The listing builds one solid part. Answer for the finished solid, in the listing's coordinates (mm). Face numbers are marked on the shaded views. A direction names the side the tool comes from. Give positions to 0.01 mm unless a question says otherwise; leave off trailing zeros. Write each loop counter-clockwise with the first axis right and the second up, starting at its lowest first coordinate (ties: lowest second). Pieces come first, ordered by that corner, then holes. Notation, with made-up numbers: (64.25, 42) -> (80.25, 42) arc R16 cw to (80.25, 69) -> close; hole circle Ø11 at (57, 29.25). An arc over 180 degrees is marked (long way). Write each question's results on one line, items separated by ' | '. Start each with the question number.
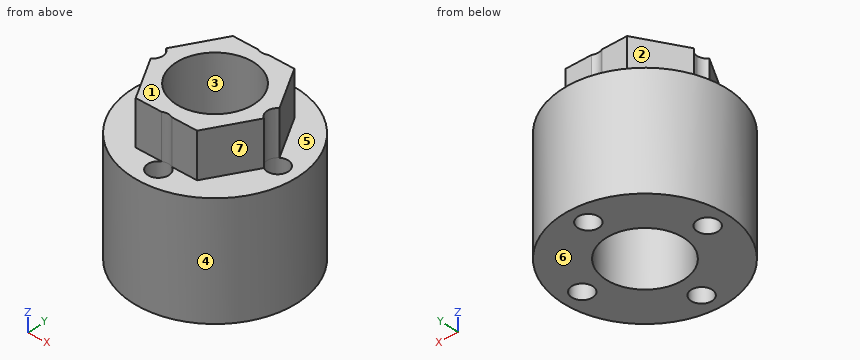
from build123d import *

# Parameters (mm, degrees)
F0_R          = 11
F1_DEPTH      = 15.2
F2_R          = 5.1
F3_DEPTH      = 50
F3_DEPTH_BACK = 50
F4_R          = 1.4
F5_DEPTH      = 25
F7_DEPTH      = 6
F8_R          = 5.2
F9_DEPTH      = 50
F10_DEPTH     = 25


with BuildPart() as f1:
    # F0 (on Top) → F1 (new body)
    with BuildSketch(Plane.XY):
        Circle(F0_R)
    extrude(amount=F1_DEPTH)

    # F2 (on face) → F3 (cut, two sides)
    with BuildSketch(Plane.XY.offset(15.2)) as f3_sk:
        Circle(F2_R)
    extrude(amount=-F3_DEPTH, mode=Mode.SUBTRACT)
    extrude(f3_sk.sketch, amount=-F3_DEPTH_BACK, mode=Mode.SUBTRACT)

    # F4 (on face) → F5 (cut)
    with BuildSketch(Plane.XY.offset(15.2)):
        with Locations((0, -8.3)):
            Circle(F4_R)
        with Locations((-8.3, 0)):
            Circle(F4_R)
        with Locations((0, 8.3)):
            Circle(F4_R)
        with Locations((8.3, 0)):
            Circle(F4_R)
    extrude(amount=-F5_DEPTH, mode=Mode.SUBTRACT)

    # F6 (on face) → F7 (join)
    with BuildSketch(Plane.XY.offset(15.2)):
        Polygon((4.039756, -7.100789), (8.169342, -0.051863), (4.129585, 7.048926), (-4.039756, 7.100789), (-8.169342, 0.051863), (-4.129585, -7.048926), align=None)
    extrude(amount=F7_DEPTH)

    # F8 (on face) → F9 (cut)
    with BuildSketch(Plane.XY.offset(21.2)):
        Circle(F8_R)
    extrude(amount=-F9_DEPTH, mode=Mode.SUBTRACT)

    # F4 (on face) → F10 (cut)
    with BuildSketch(Plane.XY.offset(15.2)):
        with Locations((-8.3, 0)):
            Circle(F4_R)
        with Locations((8.3, 0)):
            Circle(F4_R)
        with Locations((0, 8.3)):
            Circle(F4_R)
        with Locations((0, -8.3)):
            Circle(F4_R)
    extrude(amount=F10_DEPTH, mode=Mode.SUBTRACT)


solid = f1.part
1. Section B-B (z = 18) is taken. Write down the section's boundary in (x, y).
2. The mould has two halves that part along X. Classify the marked faces 1, 2, 3 and 4: pulls with the +X half, pulls with the -X half, needs draft (parallel to the pull), parting line crosses it, or undercut.
3. Section A-A (x = 0) is taken. Write down the section's boundary in (y, z).
4. Consider probe 1 along Y at (x, z) = (0, 5.25); probe 2 along Y at (x, z) = (0.5, 13); probe 3 along Z at (x, y) = (-7.5, 2.75). Determine where each line is inside the solid, lowest interval first. Write a range as [from, to].
5. Section C-C (y = 8.3) is taken. Write down the section's boundary in (x, z).
6. A tool of negligible diameter and unlimited length cuts with its end or side. For the marked faces 5, 6 and 7, from which of +Z, -Z, +X, -X, +Y, -Y can it reach the whole face along a straight path? Write none if from no direction.
7. Each of these flat-tipped pins is pushed along its axis until it touches: pin 1 Ø3 at (y, z) = (3.5, 6.5) entering from -X; pin 2 Ø2 at (y, z) = (2, 8.5) entering from -X; pin 3 Ø3 at (y, z) = (-6.5, 13) entering from -X. Where does it stop, or does it pass through?
8. Section D-D (z = 9.5) is taken. Write down the section's boundary in (x, y), then the cut area to 3 significant figures.
Results:
1) outline: (-7.52, 1.16) arc R1.4 cw to (-7.49, -1.14) -> (-4.13, -7.05) -> (-0.67, -7.07) arc R1.4 cw to (0.69, -7.08) -> (4.04, -7.1) -> (7.52, -1.16) arc R1.4 cw to (7.49, 1.14) -> (4.13, 7.05) -> (0.67, 7.07) arc R1.4 cw to (-0.69, 7.08) -> (-4.04, 7.1) -> close; hole circle Ø10.4 at (0, 0)
2) face 1: needs draft | face 2: pulls with the -X half | face 3: undercut | face 4: parting line crosses it
3) outline: (-11, 0) -> (-9.7, 0) -> (-9.7, 15.2) -> (-11, 15.2) -> close; (-6.9, 0) -> (-5.2, 0) -> (-5.2, 21.2) -> (-6.9, 21.2) -> close; (5.2, 0) -> (6.9, 0) -> (6.9, 21.2) -> (5.2, 21.2) -> close; (9.7, 0) -> (11, 0) -> (11, 15.2) -> (9.7, 15.2) -> close
4) probe 1: y = [-11, -9.7], [-6.9, -5.2], [5.2, 6.9], [9.7, 11] | probe 2: y = [-10.99, -9.61], [-6.99, -5.18], [5.18, 6.99], [9.61, 10.99] | probe 3: z = [0, 15.2]
5) outline: (-7.22, 0) -> (-1.4, 0) -> (-1.4, 15.2) -> (-7.22, 15.2) -> close; (1.4, 0) -> (7.22, 0) -> (7.22, 15.2) -> (1.4, 15.2) -> close
6) face 5: +Z | face 6: -Z, +X, -X, +Y, -Y | face 7: +Z, +X, -Y
7) pin 1: stops at x = -10.82 | pin 2: stops at x = -10.95 | pin 3: stops at x = -9.8
8) outline: circle Ø22 at (0, 0); hole circle Ø2.8 at (-8.3, 0); hole circle Ø10.4 at (0, 0); hole circle Ø2.8 at (0, -8.3); hole circle Ø2.8 at (0, 8.3); hole circle Ø2.8 at (8.3, 0) | area: 271 mm²
